Can you work these out from the model? Positions are in its coordinate system, mm. Round coordinates to 2 decimals unless told otherwise and drop trailing zeros. Order: outer loops, then holes, each group sorted by start corner. A loop starts at its lowest first (then second) coordinate and runs counter-clockwise, first axis right, second up.
Q1. If we section it at B-B (z = -4): Please give me the cut outline in (x, y), plus the area to 3 significant figures.
Q2. If we section it at D-D (z = -19): Please give me the cut outline in (x, y), plus the area to 3 significant figures.
Q3. Will these pins go through, and if not, where does the flat tip stop? P1, Ø1.5, axis at y = -0.5, z = 28, coming from the +X side; P2, Ø2, axis at y = -1.5, z = -9.5, coming from the -X side; P3, Ø2, axis at x = 3, y = -5.5, coming from the -Z side; P4, Ø4.5, axis at x = -19.05, z = 41.275, coming from the +Y side.
Q4. If we section it at C-C (y = -3.25): Count the separate pieces of the cut face and the enclosed holes in it, plus the area to 3 significant figures.
Q5. If we section it at A-A (x = -19.05): Please give me the cut outline in (y, z).
Q6. If I drill on line 1 (Z direction, x = -19, y = -3.5); line 2 (Z direction, x = 0, y = -2.5); line 3 (X direction, y = -2.75, z = 39), over which ranges is the centre line in solid material (lowest first)?
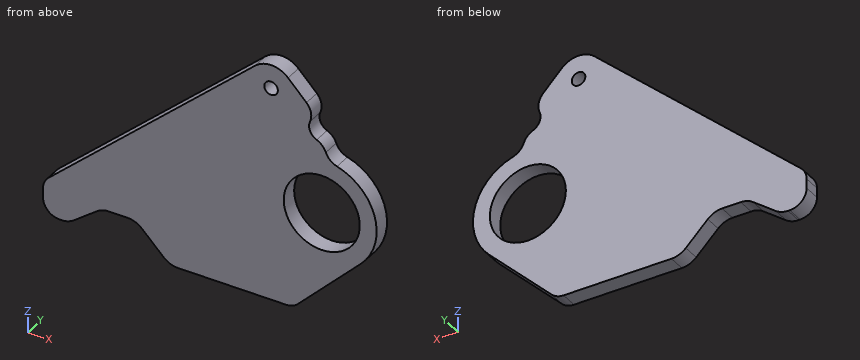
Autodesk Inventor part; units mm, degrees
ref_plane "YZ Plane" through (0, 0, 0) normal (1, 0, 0) x (0, 1, 0)
ref_plane "XZ Plane" through (0, 0, 0) normal (0, 1, 0) x (-1, 0, 0)
ref_plane "XY Plane" through (0, 0, 0) normal (0, 0, 1) x (1, 0, 0)
sketch "Sketch1" plane through (0, 0, 0) normal (0, 1, 0) x (-1, 0, 0)
  circle A0 centre (76.2, -63.1164) radius 16.7005 construction
  line L0 (69.85, -27.2929) -> (82.55, -27.2929)
  line L1 (82.55, -27.2929) -> (95.25, -36.8179)
  line L2 (95.25, -36.8179) -> (104.775, -36.8179)
  line L3 (104.775, -36.8179) -> (104.775, -24.1179)
  line L4 (104.775, -24.1179) -> (25.0156, 47.8833)
  line L5 (69.85, -27.2929) -> (57.15, -39.9929)
  line L6 (57.15, -39.9929) -> (10.8071, -39.9929)
  circle A1 centre (0, 0) radius 14.2875
  circle A2 centre (0, 0) radius 20.6375 construction
  line L7 (10.8071, -39.9929) -> (-14.5929, -14.5929)
  circle A3 centre (0, 31.75) radius 4.7625 construction
  circle A4 centre (19.05, 41.275) radius 2.5527 construction
  circle A5 centre (19.05, 41.275) radius 8.9027 construction
  line L8 (12.6625, 47.4764) -> (1.7098, 36.195)
  arc A6 (-1.27, 27.16) -> (1.7098, 36.195) centre (0, 31.75) ccw
  arc A7 (1.27, 20.5984) -> (-14.5929, -14.5929) centre (0, 0) ccw
  arc A8 (25.0156, 47.8833) -> (12.6625, 47.4764) centre (19.05, 41.275) ccw
  line L9 (-1.27, 27.16) -> (1.27, 20.5984)
  point P0 (76.2, -27.2929)
  dimension "d0" = 33.401
  dimension "d1" = 28.575
  dimension "d2" = 6.35
  dimension "d3" = 9.525
  dimension "d4" = 31.75
  dimension "d5" = 5.1054
  dimension "d6" = 6.35
  dimension "d7" = 19.05
  dimension "d8" = 9.525
  dimension "d9" = 25.4
  dimension "d10" = 25.4
  dimension "d11" = 12.7
  dimension "d12" = 12.7
  dimension "d13" = 12.7
  dimension "d15" = 76.2
  dimension "d16" = 76.2
  dimension "d17" = 12.7
  dimension "d18" = 3.175
  dimension "d19" = 9.525
  dimension "d20" = 12.7
  dimension "d34" = 4.445
  dimension "d35" = 1.27
  dimension "d36" = 1.27
extrude "Extrusion1" add sketch "Sketch1" against normal blind 6.35
fillet "Fillet1" radius 6.35 6 edges at (-1.7098, -3.175, 36.195) (-10.8071, -3.175, -39.9929) (-104.775, -3.175, -24.1179) (-104.775, -3.175, -36.8179) (1.27, -3.175, 27.16) (-1.27, -3.175, 20.5984)
fillet "Fillet2" radius 7.62 4 edges at (-69.85, -3.175, -27.2929) (-82.55, -3.175, -27.2929) (-57.15, -3.175, -39.9929) (-95.25, -3.175, -36.8179)
hole "Hole1" at (-19.05, 0, 41.275) direction (0, -1, 0) diameter 5.1054 end through all
equation "\"d17\" = d12"
properties part number "CL5-003" material "Aluminum 6061"
Solution:
1. outline: (-82.49, -6.35) - (-13.72, -6.35) - (-13.72, 0) - (-82.49, 0) - close; (13.72, -6.35) - (20.25, -6.35) - (20.25, 0) - (13.72, 0) - close
1. area: 478 mm2
2. outline: (-99.11, -6.35) - (10.19, -6.35) - (10.19, 0) - (-99.11, 0) - close
2. area: 694 mm2
3. P1: stops at x = -1.61
3. P2: stops at x = -89.69
3. P3: stops at z = -27.19
3. P4: passes through
4. separate pieces: 1
4. enclosed holes: 2
4. area: 5,850 mm2
5. outline: (-6.35, -39.99) - (0, -39.99) - (0, 38.72) - (-6.35, 38.72) - close; (-6.35, 43.83) - (0, 43.83) - (0, 50.18) - (-6.35, 50.18) - close
6. line 1: z = -39.99 to 38.72, 43.83 to 50.18
6. line 2: z = -29.19 to -14.29, 14.29 to 26.11
6. line 3: x = -34.86 to -20.21, -17.89 to -4.74
